Part print with two shaded views. Sizes in mm from the minimum x, y, z corner. Coordinates: 2 decimals unless noted, no trailing zeros. Order: outer loops, then holes, each group sorted by start corner. A loop starts at its lowest first (then second) coordinate and runs counter-clockwise, first axis right, second up. Notation, with made-up numbers: (16.5, 28.5) - (64.5, 28.5) arc R12 cw to (64.5, 50.5) - close; hole circle Ø7 at (88.5, -10). An arc over 180 degrees is marked (long way). Write each question's results on one line, items separated by ' | '. Start each with the question number.
Q1. Pin check, flat tip, straight feed: P1, Ø1.5, axis at y = 31.5, z = 5.5, coming from the +X side. Stop position of the tip, or through.
Q2. Band-saw the part on B-B, the plane x = 2.5. Write the cut outline in (y, z), then the cut area to 3 significant figures.
Q3. Band-saw the part on C-C, the plane z = 4.5. Write the cut outline in (x, y).
Q4. Band-saw the part on D-D, the plane y = 60. Write the cut outline in (x, z) (3 decimals), then the cut area to 3 significant figures.
Q5. Wall check: probe 1 along Z at (x, y) = (3.5, 16.5); probe 2 along X at (y, z) = (4, 3.25); probe 3 along X at (y, z) = (64, 2). Give the ranges that are in metal, low to high.
Q6. Band-saw the part on A-A, the plane z = 1.5. Write the cut outline in (x, y), then the cut area to 3 significant figures.
Q7. Pull direction Y, two halves, no side cores. Call the marked faces 1, 2 and 3: released by +Y, released by -Y, zero draft, split by the parting line, or undercut.
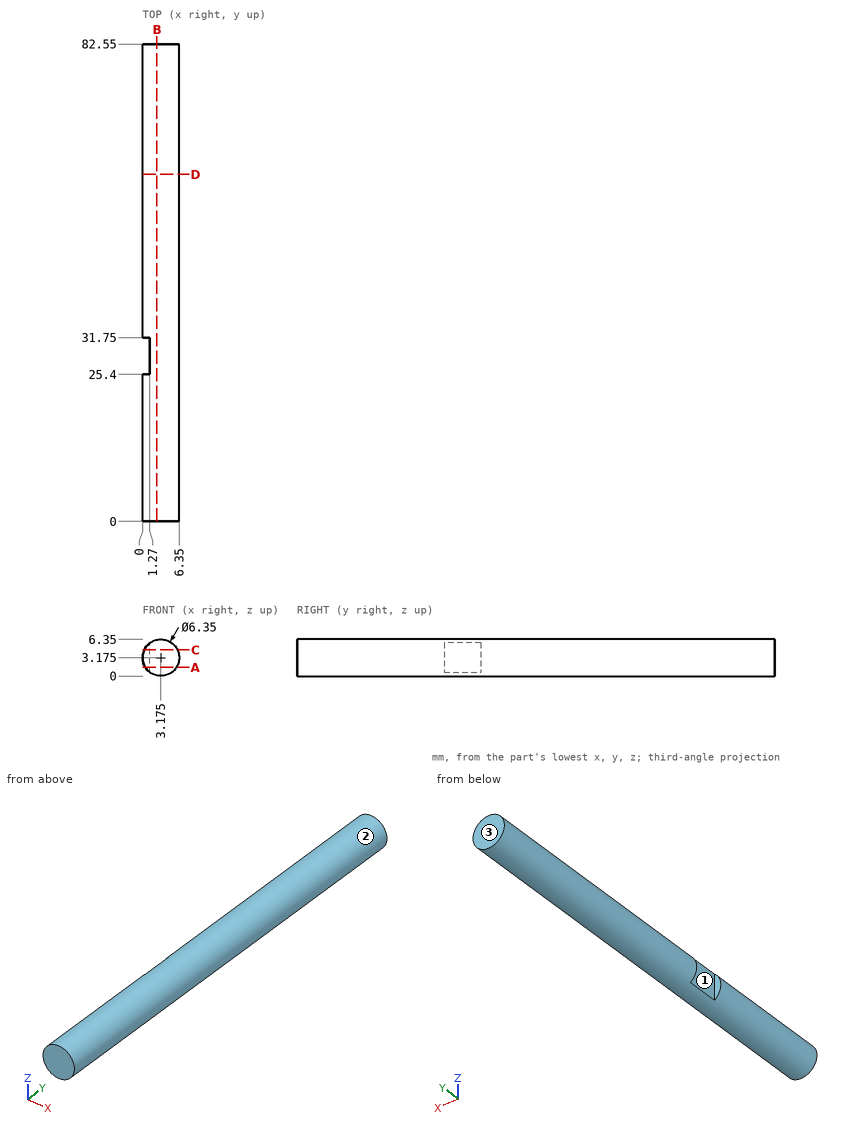
Results below:
1) P1: stops at x = 5.93
2) outline: (0, 0.07) - (82.55, 0.07) - (82.55, 6.28) - (0, 6.28) - close | area: 512 mm²
3) outline: (0.29, 0) - (6.06, 0) - (6.06, 82.55) - (0.29, 82.55) - (0.29, 31.75) - (1.27, 31.75) - (1.27, 25.4) - (0.29, 25.4) - close
4) outline: circle Ø6.35 at (3.175, 3.175) | area: 31.7 mm²
5) probe 1: z = 0.02 to 6.33 | probe 2: x = 0 to 6.35 | probe 3: x = 0.23 to 6.12
6) outline: (0.48, 0) - (5.87, 0) - (5.87, 82.55) - (0.48, 82.55) - (0.48, 31.75) - (1.27, 31.75) - (1.27, 25.4) - (0.48, 25.4) - close | area: 440 mm²
7) face 1: undercut | face 2: zero draft | face 3: released by +Y
